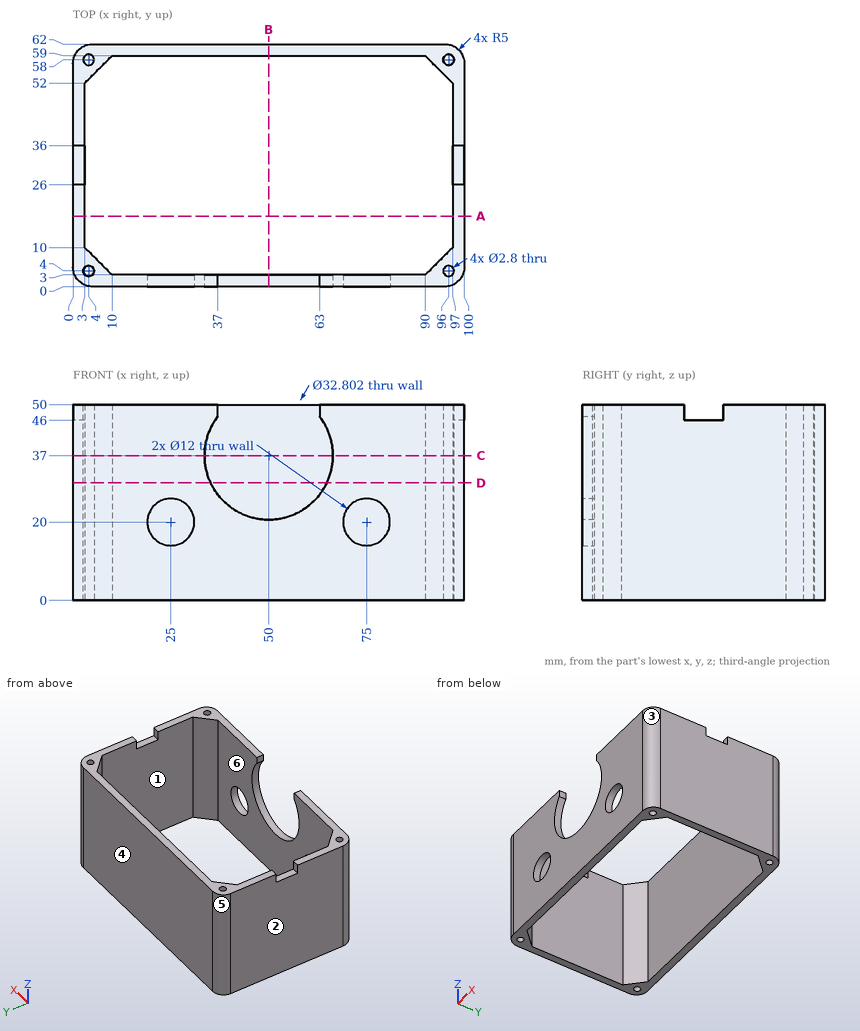
Geometry: see drawing. Coordinates: mm, zero at the bounding-box minimum. A direction names the side the tool comes from. Give positions to 0.01 mm unless a question says otherwise; leave off trailing zeros. Order: outer loops, then holes, each group sorted by start corner. A loop starts at its lowest first (then second) coordinate and runs counter-clockwise, first axis right, second up.
Q1. Section D-D on z = 30. Output: boundary loops of the cut face in (x, y).
Checked values:
outline: (0, 5) arc R5 ccw to (5, 0) - (35.17, 0) - (35.17, 3) - (10, 3) - (3, 10) - (3, 52) - (10, 59) - (90, 59) - (97, 52) - (97, 10) - (90, 3) - (64.83, 3) - (64.83, 0) - (95, 0) arc R5 ccw to (100, 5) - (100, 57) arc R5 ccw to (95, 62) - (5, 62) arc R5 ccw to (0, 57) - close; hole circle Ø2.8 at (4, 4); hole circle Ø2.8 at (4, 58); hole circle Ø2.8 at (96, 4); hole circle Ø2.8 at (96, 58)
Q2. Draft query along X for the marked faces 3, 4, 5 and 6. Return one class per face: +X half, -X half, draft (parallel to the pull), parting line (faces both ways), or undercut.
Checked values:
face 3: +X half
face 4: draft
face 5: -X half
face 6: undercut
Q3. Set-up query: the marked faces 1 and 2. Return all of +Z, -Z, +X, -X, +Y, -Y with unobstructed straight access to the full face (end or side cutting, diameter ignored); none if empty.
Checked values:
face 1: +Z, -Z
face 2: +Z, -Z, -X, +Y, -Y
Q4. Ray query, probe 1 along Y at (x, z) = (76.5, 3); probe 2 along Y at (x, z) = (96, 14); probe 3 along X at (y, z) = (11.5, 38.5). Return the intervals inside material, ascending.
Checked values:
probe 1: y = 0 to 3, 59 to 62
probe 2: y = 0.1 to 2.6, 5.4 to 9, 53 to 56.6, 59.4 to 61.9
probe 3: x = 0 to 3, 97 to 100
Q5. Section C-C on z = 37. Output: boundary loops of the cut face in (x, y).
Checked values:
outline: (0, 5) arc R5 ccw to (5, 0) - (33.6, 0) - (33.6, 3) - (10, 3) - (3, 10) - (3, 52) - (10, 59) - (90, 59) - (97, 52) - (97, 10) - (90, 3) - (66.4, 3) - (66.4, 0) - (95, 0) arc R5 ccw to (100, 5) - (100, 57) arc R5 ccw to (95, 62) - (5, 62) arc R5 ccw to (0, 57) - close; hole circle Ø2.8 at (4, 4); hole circle Ø2.8 at (4, 58); hole circle Ø2.8 at (96, 4); hole circle Ø2.8 at (96, 58)
Q6. Section A-A on y = 18. Output: boundary loops of the cut face in (x, z), and give its area (3 significant figures).
Checked values:
outline: (0, 0) - (3, 0) - (3, 50) - (0, 50) - close; (97, 0) - (100, 0) - (100, 50) - (97, 50) - close
area: 300 mm2
Q7. Contact query for flat-ended pins moving along their axis: pin 1 Ø3.5 at (x, z) = (1, 48) entering from +Y (1 decimal); pin 2 Ø1.5 at (x, z) = (99, 48.5) entering from +Y; pin 3 Ø0.9 at (y, z) = (2, 49) entering from -X. Output: stop coordinate, or through.
Checked values:
pin 1: stops at y = 61.5
pin 2: stops at y = 60.8
pin 3: stops at x = 0.7
Q8. Section B-B on x = 50. Output: boundary loops of the cut face in (y, z), and give its area (3 significant figures).
Checked values:
outline: (0, 0) - (3, 0) - (3, 20.6) - (0, 20.6) - close; (59, 0) - (62, 0) - (62, 50) - (59, 50) - close
area: 212 mm2
